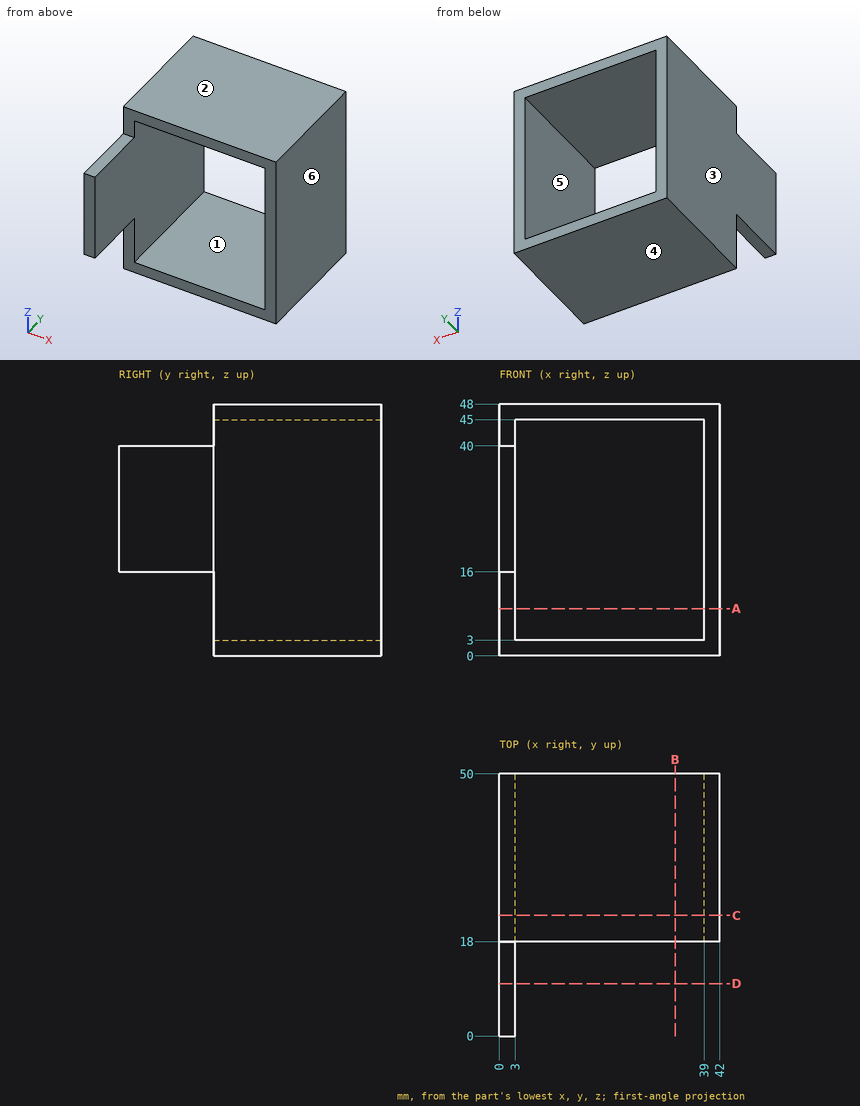
Study the drawing (mm; zero at the part's minimum x, y, z) and answer. A direction names the side the tool comes from. Give positions to 0.01 mm unless a question says otherwise; leave off trailing zeros. Loops run counter-clockwise (first coordinate to the right, second up) from the corner with the lowest first, then second, coordinate; pieces in that order, holes last. Notation, with made-up numbers: (-30.5, 37) - (6.5, 37) arc R24 cw to (6.5, 48) - close; hole circle Ø4 at (51.25, -20). An arc over 180 degrees is marked (long way). Answer in a Markdown table with one row per item. Add a question column.
Q1. A tool of negligible diameter and unlimited length cuts with its end or side. For the marked faces 1 and 2, from which of +Z, -Z, +X, -X, +Y, -Y can it reach the whole face along a straight path? Write none if from no direction.
Q2. Each of these flat-tipped pins is pushed along its axis until it touches: P1, Ø21, axis at x = 22, z = 34, coming from the -Y side; P2, Ø8, axis at x = 35, y = 33.5, coming from the -Z side; P3, Ø1.5, axis at y = 13.5, z = 34.5, coming from the +X side; P4, Ø2.5, axis at x = 2, y = 11.5, coming from the +Z side. Where does it stop, or does it pass through?
Q3. The part is cut by section B-B (x = 33.5). Determine the outline of the cut face in (y, z), and give its area (3 significant figures).
Q4. The part is cut by section C-C (y = 23). Determine the outline of the cut face in (x, z).
Q5. Consider line 1 along Z through (x, y) = (24, 36); line 2 along X through (y, z) = (24.5, 41); line 3 along X through (y, z) = (11.5, 19). Determine where each line is inside the solid, lowest interval first.
Q6. The part is cut by section A-A (z = 9). Determine the outline of the cut face in (x, y).
Q7. The part is cut by section D-D (y = 10). Determine the outline of the cut face in (x, z).
Q8. Determine the mould class of the marked faces 3, 4, 5 and 6 for opening direction X: released by +X, released by -X, zero draft, split by the parting line, or undercut.
Solution:
| question | item | result |
|---|---|---|
| 1 | face 1 | +Y, -Y |
| 1 | face 2 | +Z, +X, -X, +Y, -Y |
| 2 | P1 | passes through |
| 2 | P2 | stops at z = 0 |
| 2 | P3 | stops at x = 3 |
| 2 | P4 | stops at z = 40 |
| 3 | outline | (18, 0) - (50, 0) - (50, 3) - (18, 3) - close; (18, 45) - (50, 45) - (50, 48) - (18, 48) - close |
| 3 | area | 192 mm² |
| 4 | outline | (0, 0) - (42, 0) - (42, 48) - (0, 48) - close; hole (3, 3) - (39, 3) - (39, 45) - (3, 45) - close |
| 5 | line 1 | z = 0 to 3, 45 to 48 |
| 5 | line 2 | x = 0 to 3, 39 to 42 |
| 5 | line 3 | x = 0 to 3 |
| 6 | outline | (0, 18) - (3, 18) - (3, 50) - (0, 50) - close; (39, 18) - (42, 18) - (42, 50) - (39, 50) - close |
| 7 | outline | (0, 16) - (3, 16) - (3, 40) - (0, 40) - close |
| 8 | face 3 | released by -X |
| 8 | face 4 | zero draft |
| 8 | face 5 | undercut |
| 8 | face 6 | released by +X |
